For this review, take the finished solid that the model builds, in its own axes (mm). A direction names the side the tool comes from. Coordinates: 2 decimals unless noted, no trailing zeros. Loops run counter-clockwise (first coordinate to the right, second up) from the corner with the lowest first, then second, coordinate; pieces in that order, holes last. Notation, with made-up numbers: (20.25, 36.25) -> (79.25, 36.25) arc R20 cw to (79.25, 57.25) -> close; hole circle Ø1 at (56, 56.5). An arc over 180 degrees is marked (long way). One line per item, written item: value.
from build123d import *

# Parameters (mm, degrees)
ESQUISSE1_R        = 2
ESQUISSE1_W        = 5
ESQUISSE1_H        = 5
BOSS_EXTRU_1_DEPTH = 5
CONG_1_R           = 5


with BuildPart() as part:
    # Esquisse1 → Boss.-Extru.1 (new body)
    with BuildSketch(Plane.XY):
        Polygon((0, 37.65), (71, 37.65), (71, -37.65), (0, -37.65), (0, -25), (-35, -25), (-35, -10), (-5, -10), (-5, 10), (-35, 10), (-35, 25), (0, 25), align=None)
        with Locations((-30, 17.5)):
            Circle(ESQUISSE1_R, mode=Mode.SUBTRACT)
        with Locations(Location((-30, -17.5, 0), (0, 0, 180))):
            Circle(ESQUISSE1_R, mode=Mode.SUBTRACT)
        with Locations((36, 33.15)):
            Circle(ESQUISSE1_R, mode=Mode.SUBTRACT)
        with Locations(Location((36, -33.15, 0), (0, 0, 90))):
            Circle(ESQUISSE1_R, mode=Mode.SUBTRACT)
        with Locations((28.5, 33.15)):
            Rectangle(ESQUISSE1_W, ESQUISSE1_H, mode=Mode.SUBTRACT)
        with Locations((43.5, 33.15)):
            Rectangle(ESQUISSE1_W, ESQUISSE1_H, mode=Mode.SUBTRACT)
        with Locations((28.5, -33.15)):
            Rectangle(ESQUISSE1_W, ESQUISSE1_H, mode=Mode.SUBTRACT)
        with Locations((43.5, -33.15)):
            Rectangle(ESQUISSE1_W, ESQUISSE1_H, mode=Mode.SUBTRACT)
    extrude(amount=BOSS_EXTRU_1_DEPTH)

    # Congé1
    cong_1_edges = [part.edges().sort_by_distance(p)[0] for p in [
        (-35, -10, 2.5),
        (-35, 10, 2.5),
        (-35, 25, 2.5),
        (-35, -25, 2.5),
    ]]
    fillet(cong_1_edges, radius=CONG_1_R)


solid = part.part
1. Take a section at C-C, the plane y = -33.15. Give the boundary of the cut face in (x, z), and give its area (3 significant figures).
Return value:
outline: (0, 0) -> (26, 0) -> (26, 5) -> (0, 5) -> close; (31, 0) -> (34, 0) -> (34, 5) -> (31, 5) -> close; (38, 0) -> (41, 0) -> (41, 5) -> (38, 5) -> close; (46, 0) -> (71, 0) -> (71, 5) -> (46, 5) -> close
area: 285 mm2
2. For faces 5 (the flat face through (35, 37.65, 2)), 6 (the cylindrical face through (-33, -24, 3)), 7 (the flat face through (-15, 25, 2)), 8 (the cylindrical face through (-34, 12, 3)), 9 (the flat face through (41, 33, 2)), list the 3-axis set-ups (+Z, -Z, +X, -X, +Y, -Y) from which the entire face can be reached by the end or side of a thin tool; tool diameter is ignored.
Return value:
face 5: +Z, -Z, +X, -X, +Y
face 6: +Z, -Z, -X, -Y
face 7: +Z, -Z, -X, +Y
face 8: +Z, -Z, -X
face 9: +Z, -Z
3. Take a section at B-B, the plane x = 36. Give the boundary of the cut face in (y, z).
Return value:
outline: (-37.65, 0) -> (-35.15, 0) -> (-35.15, 5) -> (-37.65, 5) -> close; (-31.15, 0) -> (31.15, 0) -> (31.15, 5) -> (-31.15, 5) -> close; (35.15, 0) -> (37.65, 0) -> (37.65, 5) -> (35.15, 5) -> close
4. To check wall thickness, follow probe 1 along Y at (x, z) = (36, 3.8); probe 2 along Y at (x, z) = (28, 2.95); probe 3 along X at (y, z) = (-33.15, 2.1). State the ranges of each line that lie inside material, in increasing order. Write a range as from..to.
Return value:
probe 1: y = -37.65..-35.15, -31.15..31.15, 35.15..37.65
probe 2: y = -37.65..-35.65, -30.65..30.65, 35.65..37.65
probe 3: x = 0..26, 31..34, 38..41, 46..71
5. The part is to be moulded in two halves that separate along X. For faces 1 (the flat face through (28, 30.65, 2)), 2 (the flat face through (43, 35.65, 2)), 3 (the flat face through (0, -31, 2)), 4 (the flat face through (71, 1, 2)), say which applies: pulls with the +X half, pulls with the -X half, needs draft (parallel to the pull), parting line crosses it, or undercut.
Return value:
face 1: undercut
face 2: undercut
face 3: pulls with the -X half
face 4: pulls with the +X half
6. Take a section at A-A, the plane y = -17.5. Give the boundary of the cut face in (x, z), and give its area (3 significant figures).
Return value:
outline: (-35, 0) -> (-32, 0) -> (-32, 5) -> (-35, 5) -> close; (-28, 0) -> (71, 0) -> (71, 5) -> (-28, 5) -> close
area: 510 mm2
7. Insertion check: pin 1 Ø1.5 at (y, z) = (-34, 2.5) entering from -X; pin 2 Ø2.5 at (x, z) = (-13.5, 2.5) entering from -Y; pin 3 Ø1 at (y, z) = (-24, 4.5) entering from -X. Each pin has a flat end and moves straight along its axis. Give the tip position at first contact, or say it passes through.
Return value:
pin 1: stops at x = 0
pin 2: stops at y = -25
pin 3: stops at x = -33.57
8. Take a section at D-D, the plane z = 2.3. Give the number of separate pieces and of enclosed holes in the cut face, and give its area (3 significant figures).
Return value:
separate pieces: 1
enclosed holes: 8
area: 6,320 mm2
